Geometry: see drawing. Coordinates: mm, zero at the bounding-box minimum. Coordinates: 2 decimals unless noted, no trailing zeros. Loops run counter-clockwise (first coordinate to the right, second up) from the corner with the lowest first, then second, coordinate; pieces in that order, holes last. Notation, with made-up numbers: (66.25, 8.25) - (83.25, 8.25) arc R16 ccw to (83.25, 27.25) - close; hole circle Ø1 at (86, 13.5). An arc over 180 degrees is marked (long way). Use one line per item in the form item = value.
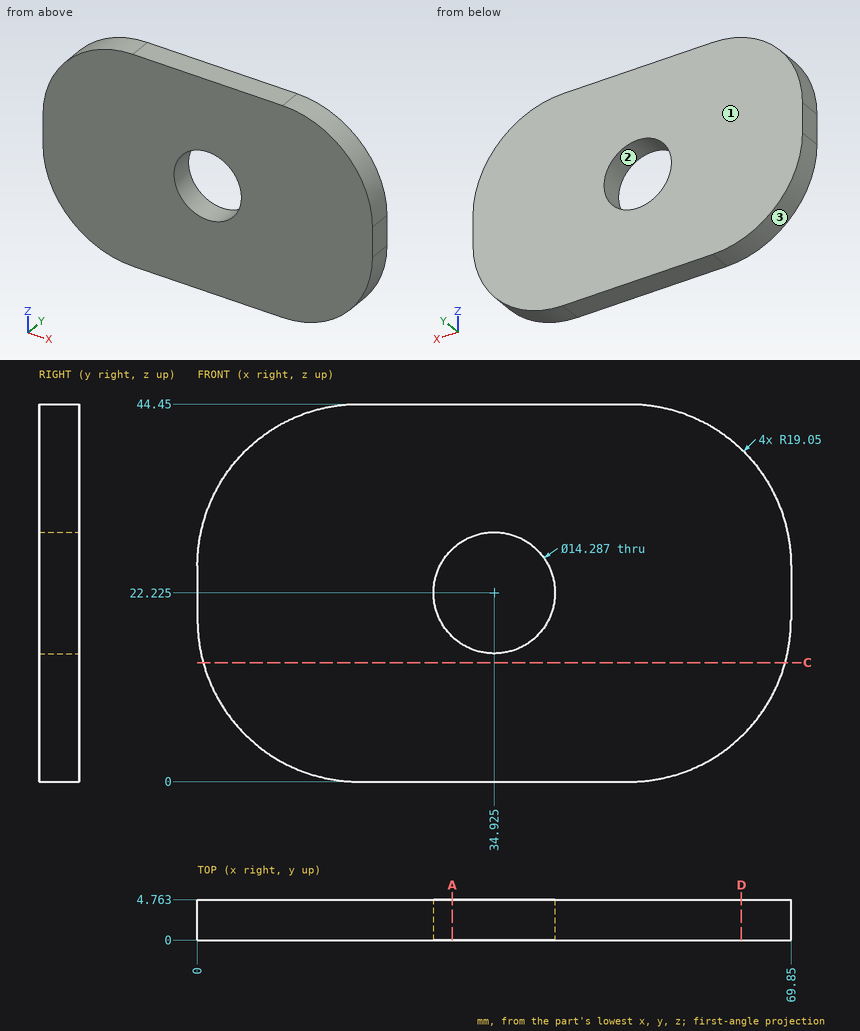
Q1. Cut plane A-A, the plane x = 30. Return loops of the section in (y, z), then the cut area to 3 significant figures.
Check values:
outline = (0, 0) - (4.76, 0) - (4.76, 17.05) - (0, 17.05) - close; (0, 27.4) - (4.76, 27.4) - (4.76, 44.45) - (0, 44.45) - close
area = 162 mm²
Q2. Cut plane C-C, the plane z = 14. Return loops of the section in (x, y), then the cut area to 3 significant figures.
Check values:
outline = (0.68, 0) - (69.17, 0) - (69.17, 4.76) - (0.68, 4.76) - close
area = 326 mm²
Q3. Ray query, line 1 along Z through (x, y) = (36, 1.3); line 2 along Z through (x, y) = (51.5, 0.3); line 3 along X through (y, z) = (3.3, 35) (1 decimal). Return the intervals inside material, ascending. Write a range as [from, to].
Check values:
line_1 = [0, 15.16], [29.29, 44.45]
line_2 = [0.01, 44.44]
line_3 = [2.6, 67.3]
Q4. Pull-direction query (X, two-part tool) for the marked faces 1, 2 and 3; classes: pulls with the +X half, pulls with the -X half, needs draft (parallel to the pull), parting line crosses it, or undercut.
Check values:
face_1 = needs draft
face_2 = undercut
face_3 = pulls with the -X half
Q5. Cut plane D-D, the plane x = 64. Return loops of the section in (y, z) (1 decimal), then the cut area to 3 significant figures.
Check values:
outline = (0, 5.3) - (4.8, 5.3) - (4.8, 39.1) - (0, 39.1) - close
area = 161 mm²
Q6. First-contact query: P1, Ø2, axis at x = 10.5, y = 1.5, coming from the +Z side. Flat tip, straight axial feed; report the tip coordinate or a pass-through.
Check values:
P1 = 42.89
